Could you check a few things on this drawing? It's one solid part, dimensions in mm from its lowest x, y, z. Give positions to 0.01 mm unless a question says otherwise; leave off trailing zeros. Order: outer loops, then holes, each group sorted by start corner. A loop starts at its lowest first (then second) coordinate and runs counter-clockwise, first axis right, second up. Notation, with made-up numbers: M -27.75,-13 L 3.25,-13 A19 ccw 3.25,2 Z; hole C 53,-12 d10. An arc over 180 degrees is marked long. Use one line per item in the form item = value.
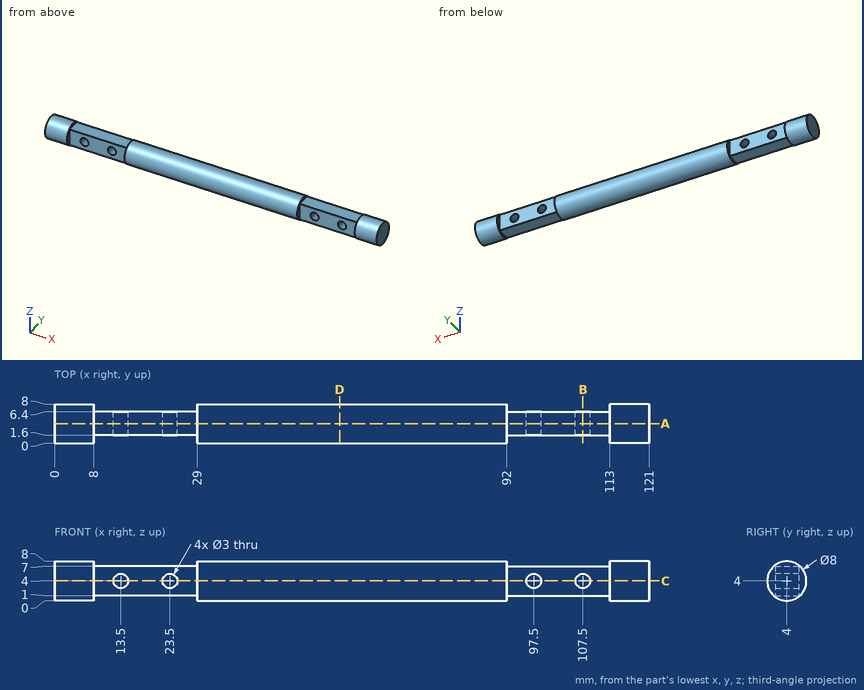
Q1. I need wall thicknesses on L1, parallel to X at y = 3.25, z = 7.75; L2, parallel to X at y = 4.25, z = 4; L3, parallel to Z at x = 77, y = 4.25. Which ranges of each line are inside material? Lowest first, please.
Found:
L1 = 0 to 8, 29 to 92, 113 to 121
L2 = 0 to 12, 15 to 22, 25 to 96, 99 to 106, 109 to 121
L3 = 0.01 to 7.99
Q2. I want a section at C-C on z = 4. State how many separate pieces and enclosed holes the cut face has, then the cut area to 3 significant figures.
Found:
separate_pieces = 5
enclosed_holes = 0
area = 776 mm²
Q3. I'm going to push flat-ended pins straight in: pin 1 Ø4 at (x, z) = (13.5, 4) entering from -Y; pin 2 Ø4 at (x, y) = (15, 4.5) entering from +Z; pin 3 Ø1 at (x, y) = (12.5, 6.5) entering from -Z. Where does each tip first touch, or does it pass through?
Found:
pin_1 = 1.6
pin_2 = 7
pin_3 = 1
Q4. I want a section at B-B on x = 107.5. Write out the boundary of the cut face in (y, z).
Found:
outline = M 1.6,1 L 6.4,1 L 6.4,2.5 L 1.6,2.5 Z; M 1.6,5.5 L 6.4,5.5 L 6.4,7 L 1.6,7 Z
Q5. I want a section at A-A on y = 4. Write out the boundary of the cut face in (x, z).
Found:
outline = M 0,0 L 8,0 L 8,1 L 29,1 L 29,0 L 92,0 L 92,1 L 113,1 L 113,0 L 121,0 L 121,8 L 113,8 L 113,7 L 92,7 L 92,8 L 29,8 L 29,7 L 8,7 L 8,8 L 0,8 Z; hole C 13.5,4 d3; hole C 23.5,4 d3; hole C 97.5,4 d3; hole C 107.5,4 d3
Q6. I want a section at D-D on x = 58. Write out the boundary of the cut face in (y, z), then the cut area to 3 significant figures.
Found:
outline = C 4,4 d8
area = 50.3 mm²
